Check sheet for the drawn part. Datum: minimum x, y, z corner. Units: mm. A direction names the side the tool comes from. Round coordinates to 2 decimals unless told otherwise and drop trailing zeros. Write each loop counter-clockwise with the first axis right and the second up, starting at its lowest first coordinate (ties: lowest second). Pieces come first, ordered by that corner, then holes. Notation, with made-up numbers: (73, 15.5) -> (127, 15.5) arc R22 cw to (127, 41.5) -> close; hole circle Ø10 at (14.25, 8.25). An arc over 180 degrees is marked (long way). Use a Markdown table: item, result.
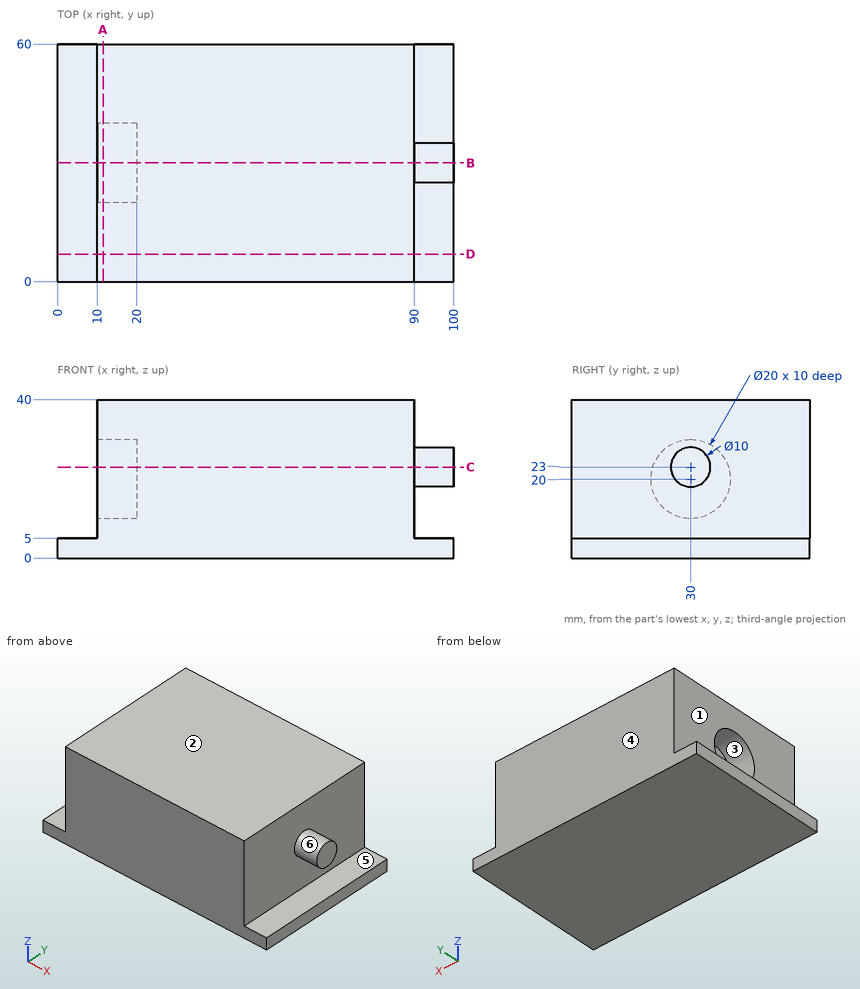
(1) Gauge pin test, flat ends, axial feed: pin 1 Ø10 at (y, z) = (39, 18.5) entering from -X; pin 2 Ø4 at (y, z) = (20, 15) entering from +X; pin 3 Ø3 at (x, y) = (95, 22.5) entering from +Z. Record the tip position at first contact, or that the pin passes through.
A:
| item | result |
|---|---|
| pin 1 | stops at x = 10 |
| pin 2 | stops at x = 90 |
| pin 3 | stops at z = 5 |
(2) Section check B-B on y = 30. Record the cut outline in (x, z), plus the area to 3 significant figures.
A:
| item | result |
|---|---|
| outline | (0, 0) -> (100, 0) -> (100, 5) -> (90, 5) -> (90, 18) -> (100, 18) -> (100, 28) -> (90, 28) -> (90, 40) -> (10, 40) -> (10, 30) -> (20, 30) -> (20, 10) -> (10, 10) -> (10, 5) -> (0, 5) -> close |
| area | 3,200 mm2 |
(3) Section check A-A on x = 11.5. Record the cut outline in (y, z), plus the area to 3 significant figures.
A:
| item | result |
|---|---|
| outline | (0, 0) -> (60, 0) -> (60, 40) -> (0, 40) -> close; hole circle Ø20 at (30, 20) |
| area | 2,090 mm2 |
(4) Section check D-D on y = 7. Record the cut outline in (x, z).
A:
| item | result |
|---|---|
| outline | (0, 0) -> (100, 0) -> (100, 5) -> (90, 5) -> (90, 40) -> (10, 40) -> (10, 5) -> (0, 5) -> close |
(5) Thickness scan on line 1 (Y direction, x = 17.5, z = 20); line 2 (X direction, y = 35, z = 31); line 3 (X direction, y = 32, z = 17.5). Record the ranges inside material, lowest first.
A:
| item | result |
|---|---|
| line 1 | y = 0 to 20, 40 to 60 |
| line 2 | x = 10 to 90 |
| line 3 | x = 20 to 90 |
(6) Release check for a two-part mould opening along Y. For the marked faces 3, 4, 5 and 6 record: +Y half, -Y half, draft (parallel to the pull), parting line (faces both ways), or undercut.
A:
| item | result |
|---|---|
| face 3 | undercut |
| face 4 | +Y half |
| face 5 | draft |
| face 6 | parting line |
(7) Access from +Z, -Z, +X, -X, +Y, -Y to the whole of each face (thin tool, end or side, straight path). Record for the marked faces 1 and 2.
A:
| item | result |
|---|---|
| face 1 | +Z, -X, +Y, -Y |
| face 2 | +Z, +X, -X, +Y, -Y |
(8) Section check C-C on z = 23. Record the cut outline in (x, y).
A:
| item | result |
|---|---|
| outline | (10, 0) -> (90, 0) -> (90, 25) -> (100, 25) -> (100, 35) -> (90, 35) -> (90, 60) -> (10, 60) -> (10, 39.54) -> (20, 39.54) -> (20, 20.46) -> (10, 20.46) -> close |
